Autodesk Inventor part; units mm, degrees
ref_plane "YZ Plane" through (0, 0, 0) normal (1, 0, 0) x (0, 1, 0)
ref_plane "XZ Plane" through (0, 0, 0) normal (0, 1, 0) x (-1, 0, 0)
ref_plane "XY Plane" through (0, 0, 0) normal (0, 0, 1) x (1, 0, 0)
sketch "Sketch1" plane through (0, 0, 0) normal (0, 1, 0) x (-1, 0, 0)
  circle A0 centre (0, 0) radius 1.4
  dimension "d0" = 2.8
sketch "Sketch2" plane through (0, 0, 0) normal (0, 1, 0) x (-1, 0, 0)
  point P0 (0, 0)
extrude "Extrusion1" add sketch "Sketch1" along normal blind 7
sketch "Sketch3" plane through (0, 7, 0) normal (0, 1, 0) x (1, 0, 0)
  line L0 (1.8253, 0.7457) -> (1.818, -0.7634)
  line L1 (1.818, -0.7634) -> (0.7457, -1.8253)
  line L2 (0.7457, -1.8253) -> (-0.7634, -1.818)
  line L3 (-0.7634, -1.818) -> (-1.8253, -0.7457)
  line L4 (-1.8253, -0.7457) -> (-1.818, 0.7634)
  line L5 (-1.818, 0.7634) -> (-0.7457, 1.8253)
  line L6 (-0.7457, 1.8253) -> (0.7634, 1.818)
  line L7 (0.7634, 1.818) -> (1.8253, 0.7457)
  line L8 (-1.8216, 0.0088) -> (1.8216, -0.0088) construction
  line L9 (-0.0088, -1.8216) -> (0.0088, 1.8216) construction
  point P0 (0, 0)
  point P1 (0, 0)
  point P2 (0, 0)
  point P3 (0, 0)
extrude "Extrusion2" add sketch "Sketch3" along normal blind 2
sketch "Sketch4" plane through (-0.7457, 7, -1.8253) normal (0.0048553, 0, -0.9999882) x (-0.9999882, 0, -0.0048553)
  line L0 (-1.5091, 2) -> (0, 2)
  line L1 (0, 2) -> (0, 0)
  line L2 (0, 0) -> (-1.5091, 0)
  line L3 (-1.5091, 0) -> (-1.5091, 2)
  point P0 (-0.7546, -7)
extrude "Extrusion3" add sketch "Sketch4" along normal blind 10
sketch "Sketch5" plane through (0, 9, 0) normal (0, 1, 0) x (1, 0, 0)
  point P0 (0, 0)
sketch "Sketch6" plane through (0, 9, 0) normal (0, 1, 0) x (1, 0, 0)
  point P0 (0, 0)
thread "Thread1"
sketch "Sketch7" plane through (0, 9, 0) normal (0, 1, 0) x (1, 0, 0)
  circle A0 centre (0.062, 12.7642) radius 1.2414
  point P0 (0, 0)
extrude "Extrusion4" add sketch "Sketch7" against normal blind 2
sketch "Sketch8" plane through (0, 9, 0) normal (0, 1, 0) x (1, 0, 0)
  point P0 (0, 0)
sketch "Sketch9" plane through (0, 9, 0) normal (0, 1, 0) x (1, 0, 0)
  point P0 (0, 0)
sketch "Sketch10" plane through (0, 9, 0) normal (0, 1, 0) x (1, 0, 0)
  line L0 (10.3239, 13.7463) -> (10.3549, 13.7463)
  point P0 (0, 0)
extrude "Extrusion5" [suppressed]
sketch "Sketch11" plane through (0, 9, 0) normal (0, 1, 0) x (1, 0, 0)
  point P0 (0, 0)
sketch "Sketch12" plane through (0, 9, 0) normal (0, 1, 0) x (1, 0, 0)
  point P0 (0, 0)
sketch "Sketch13" plane through (0, 9, 0) normal (0, 1, 0) x (1, 0, 0)
  line L0 (0.062, 11.5229) -> (9.5019, 11.5229)
  line L1 (0.062, 11.5229) -> (0.062, 14.0056)
  arc A0 (0.8117, 11.7749) -> (-0.6974, 11.7822) centre (0.062, 12.7642) ccw
  line L2 (0.062, 14.0056) -> (9.5019, 14.0056)
  line L3 (9.5019, 11.5229) -> (9.5019, 14.0056)
  point P0 (0, 0)
extrude "Extrusion6" add sketch "Sketch13" against normal blind 2
sketch "Sketch14" plane through (0, 9, 0) normal (0, 1, 0) x (1, 0, 0)
  line L0 (9.5019, 14.0056) -> (9.5019, 11.5229)
  circle A0 centre (9.5019, 12.7642) radius 1.2415
  point P0 (0, 0)
  dimension "d17" = 2.483
extrude "Extrusion7" add sketch "Sketch14" against normal blind 2
sketch "Sketch15" plane through (0, 9, 0) normal (0, 1, 0) x (1, 0, 0)
  arc A0 (9.4834, 11.5229) -> (9.4834, 14.0056) centre (9.5019, 12.7642) ccw
  line L0 (10.7434, 12.7642) -> (13.7224, 9.3009)
  line L1 (9.4834, 11.5229) -> (11.3674, 9.2776)
  line L2 (9.4834, 11.5229) -> (12.4144, 11.5229) construction
  arc A1 (11.3674, 9.2776) -> (13.7224, 9.3009) centre (12.5353, 10.2576) ccw
  point P0 (0, 0)
  dimension "d20" = 50
extrude "Extrusion8" add sketch "Sketch15" against normal blind 2
fillet "Fillet1" radius 2 1 edges at (0.8105, 8, -11.5229)
fillet "Fillet2" radius 2 1 edges at (9.5019, 8, -11.5229)
fillet "Fillet3" radius 2 1 edges at (10.7434, 8, -12.7642)
properties part number "Servo_Arm_Hook_M"
Build history of the part. All positions in model axes, mm. A direction names the side the tool comes from. Give positions to 0.01 mm unless a question says otherwise; leave off trailing zeros. Loops run counter-clockwise (first coordinate to the right, second up) from the corner with the lowest first, then second, coordinate; pieces in that order, holes last. Notation, with made-up numbers: (-38, 10) -> (14, 10) arc R23 ccw to (14, 49) -> close; hole circle Ø4 at (-25, -38). An arc over 180 degrees is marked (long way). Answer in a Markdown table with one row per item.
Item 1: Slice it at B-B on z = -9. Write the cut outline in (x, y).
Findings below:
| item | result |
|---|---|
| outline | (-0.71, 7) -> (0.8, 7) -> (0.8, 9) -> (-0.71, 9) -> close; (11.67, 7) -> (13.4, 7) -> (13.4, 9) -> (11.67, 9) -> close |
Item 2: Flat gauge pins, fed straight in: P1, Ø0.6, axis at x = 10, z = -13.5, coming from the -Y side; P2, Ø1.6, axis at x = 5.5, y = 8, coming from the +Z side; P3, Ø3, axis at x = 9.5, z = -11, coming from the +Y side; P4, Ø3, axis at x = 4, y = 2.5, coming from the +Z side. Where does each tip first touch, or does it go through?
Findings below:
| item | result |
|---|---|
| P1 | stops at y = 7 |
| P2 | stops at z = -11.52 |
| P3 | stops at y = 9 |
| P4 | passes through |
Item 3: Probe line 1 along Y through (x, z) = (0.25, -5.75); line 2 along Z through (x, y) = (1.75, 7.5); line 3 along X through (y, z) = (6.5, 0.75). List the from-to ranges inside material, lowest first. Write a range as [from, to].
Findings below:
| item | result |
|---|---|
| line 1 | y = [7, 9] |
| line 2 | z = [-14.01, -11.22], [-0.82, 0.83] |
| line 3 | x = [-1.18, 1.18] |
Item 4: Tool access for faces 1 (the cylindrical face through (1.37, 7.99, -10.92)), 2 (the flat face through (10.72, 8.01, -10.05)), 3 (the cylindrical face through (1.4, 3.45, -0.06)): list every direction of +Z, -Z, +X, -X, +Y, -Y with a clear straight run to the whole face (end or side of a thin tool).
Findings below:
| item | result |
|---|---|
| face 1 | +Y, -Y |
| face 2 | +Z, +Y, -Y |
| face 3 | -Y |
Item 5: Mould opens along Z. For faces 4 (the cylindrical face through (10.259, 8.014, -13.748)), 5 (the flat face through (-1.287, 7.986, 1.289)), 6 (the cylindrical face through (-1.1, 8, -13.2)), 7 (the flat face through (1.287, 7.986, -1.289)) say: pulls with the +Z half, pulls with the -Z half, needs draft (parallel to the pull), parting line crosses it, or undercut.
Findings below:
| item | result |
|---|---|
| face 4 | pulls with the -Z half |
| face 5 | pulls with the +Z half |
| face 6 | undercut |
| face 7 | undercut |
Item 6: Slice it at A-A on y = 7.75. Write the cut outline in (x, z).
Findings below:
| item | result |
|---|---|
| outline | (-1.83, 0.75) -> (-1.82, -0.76) -> (-0.75, -1.83) -> (-0.7, -11.78) arc R1.24 ccw to (0.06, -14.01) -> (9.5, -14.01) arc R1.24 ccw to (10.7, -13.1) arc R2 cw to (11.1, -12.34) -> (13.72, -9.3) arc R1.52 ccw to (11.37, -9.28) -> (10.08, -10.81) arc R2 cw to (8.55, -11.52) -> (2.8, -11.52) arc R2 cw to (0.8, -9.53) -> (0.76, -1.82) -> (1.83, -0.75) -> (1.82, 0.76) -> (0.75, 1.83) -> (-0.76, 1.82) -> close |
Item 7: Slice it at C-C on z = 0. Write the cut outline in (x, y), plus the area to 3 significant figures.
Findings below:
| item | result |
|---|---|
| outline | (-1.82, 7) -> (-1.4, 7) -> (-1.4, 0) -> (1.4, 0) -> (1.4, 7) -> (1.82, 7) -> (1.82, 9) -> (-1.82, 9) -> close |
| area | 26.9 mm² |
Item 8: Slice it at D-D on x = 7.5. Write the cut outline in (y, z).
Findings below:
| item | result |
|---|---|
| outline | (7, -14.01) -> (9, -14.01) -> (9, -11.52) -> (7, -11.52) -> close |
